Geometry check sheet. Reference: the model listing, model coordinates, mm. A direction names the side the tool comes from. Coordinates: 2 decimals unless noted, no trailing zeros. Loops run counter-clockwise (first coordinate to the right, second up) from the corner with the lowest first, then second, coordinate; pieces in that order, holes last.
from build123d import *

# Parameters (mm, degrees)
F0_W     = 1016
F0_H     = 762
F1_DEPTH = 762
F2_SIZE  = 50.8
F3_R     = 63.5
F3_R_2   = 76.2
F4_DEPTH = 474.98
F6_DEPTH = 254
F7_R     = 25.4


with BuildPart() as f1:
    # F0 (on Top) → F1 (new body)
    with BuildSketch(Plane.XY):
        Rectangle(F0_W, F0_H)
    extrude(amount=F1_DEPTH)

    # F2
    f2_edges = [f1.edges().sort_by_distance(p)[0] for p in [
        (0, -381, 762),
        (508, 0, 762),
        (0, 381, 762),
        (-508, 0, 762),
    ]]
    chamfer(f2_edges, length=F2_SIZE)

    # F3 (on face) → F4 (cut)
    with BuildSketch(Plane.XY.offset(762)):
        with Locations((254, 154.278123)):
            Circle(F3_R)
        with Locations((160.084128, -127)):
            Circle(F3_R_2)
        with Locations((-190.5, 161.287912)):
            Circle(F3_R)
        with Locations((-248.486163, -203.2)):
            Circle(F3_R_2)
    extrude(amount=-F4_DEPTH, mode=Mode.SUBTRACT)

    # F5 (on face) → F6 (cut)
    with BuildSketch(Plane.YZ.offset(508)):
        Polygon((-172.04284, 448.87892), (-172.04284, 321.87892), (78.168072, 321.87892), (78.168072, 575.87892), (-48.828607, 576.797382), (-45.043587, 448.443412), align=None)
    extrude(amount=-F6_DEPTH, mode=Mode.SUBTRACT)

    # F7
    f7_edges = [f1.edges().sort_by_distance(p)[0] for p in [
        (254, -108.543213, 448.661166),
        (254, -46.936097, 512.620397),
        (254, 14.669732, 576.338151),
        (254, 78.168072, 448.87892),
        (254, -46.937384, 321.87892),
        (254, -172.04284, 385.37892),
    ]]
    fillet(f7_edges, radius=F7_R)


solid = f1.part
1) Access from +Z, -Z, +X, -X, +Y, -Y to the whole of each face (thin tool, end or side, straight path). Record for faces 1 (the flat face through (395, -172.043, 386)), 2 (the cylindrical face through (232.765, -104.112, 527.835)), 3 (the flat face through (-6, 5, 762)).
Data:
face 1: +X
face 2: +Z
face 3: +Z, +X, -X, +Y, -Y
2) Section check A-A on x = -208. Record the cut outline in (y, z), and give its area (3 significant figures).
Data:
outline: (-381, 0) - (381, 0) - (381, 711.2) - (330.2, 762) - (222.33, 762) - (222.33, 287.02) - (100.25, 287.02) - (100.25, 762) - (-138.65, 762) - (-138.65, 287.02) - (-267.75, 287.02) - (-267.75, 762) - (-330.2, 762) - (-381, 711.2) - close
area: 459,000 mm2
3) Material ranges on probe 1 along Y at (x, z) = (420, 366); probe 2 along Y at (x, z) = (-211, 384.5); probe 3 along X at (y, z) = (-174, 714), recorded low to high.
Data:
probe 1: y = -381 to -172.04, 78.17 to 381
probe 2: y = -381 to -269.54, -136.86 to 101.19, 221.39 to 381
probe 3: x = -505.2 to -318.87, -178.1 to 100.11, 220.06 to 505.2
4) Mould release check, pull along X, two halves, no side actions. Record for faces 4 (the flat face through (395, -49, 321.879)), 5 (the cylindrical face through (261.638, 70.925, 450.657)), 6 (the flat face through (-250, -202, 287.02)): +X half, -X half, draft (parallel to the pull), parting line (faces both ways), or undercut.
Data:
face 4: draft
face 5: +X half
face 6: undercut
5) Section check B-B on z = 512. Count the separate pieces of the cut face and the enclosed holes in it, and give its area (3 significant figures).
Data:
separate pieces: 1
enclosed holes: 4
area: 681,000 mm2
